Can you work these out from the drawing? Everything is in mm from the part's minimum corner. A direction names the side the tool comes from. Give positions to 0.01 mm unless a question says otherwise; leave off trailing zeros. Order: outer loops, then holes, each group sorted by start corner. A loop starts at its lowest first (then second) coordinate and runs counter-clockwise, first axis right, second up. Notation, with made-up numbers: M -33.5,74.5 L 7.5,74.5 A28 ccw 7.5,99.5 Z; hole C 47,67 d1. An arc over 180 degrees is marked long. Use a Markdown table: item, result. Add a question column.
Item 1: If I drill on L1, parallel to X at y = 1.55, z = 19.05; L2, parallel to Y at x = 24, z = 11.5; L3, parallel to Y at x = 5, z = 31.5, over which ranges is the centre line in solid material (lowest first)? Write a range as from..to.
Item 2: Suppose I cut it at D-D on x = 6.5. Write out the boundary of the cut face in (y, z).
Item 3: Suppose I cut it at B-B on y = 7.5. Write out the boundary of the cut face in (x, z).
Item 4: Suppose I cut it at C-C on z = 4. Write out the boundary of the cut face in (x, y).
Item 5: For the marked faces 4, 5 and 6, which set-ups out of +Z, -Z, +X, -X, +Y, -Y let a thin tool reach every point of the face, with its end or its side?
Item 6: I'm going to push flat-ended pins straight in: pin 1 Ø1 at (y, z) = (3, 4.5) entering from -X (1 decimal); pin 2 Ø1.5 at (x, z) = (6, 16) entering from -Y; pin 3 Ø3.5 at (x, y) = (20, 9.5) entering from +Z. Where does each tip first touch, or does it pass through?
Item 7: Suppose I cut it at A-A on x = 19.05. Write out the boundary of the cut face in (y, z).
Item 8: If we mould it in two halves opening along X, with no side actions, what happens to the marked faces 1, 2 and 3? For each: released by +X, released by -X, zero draft, split by the parting line, or undercut.
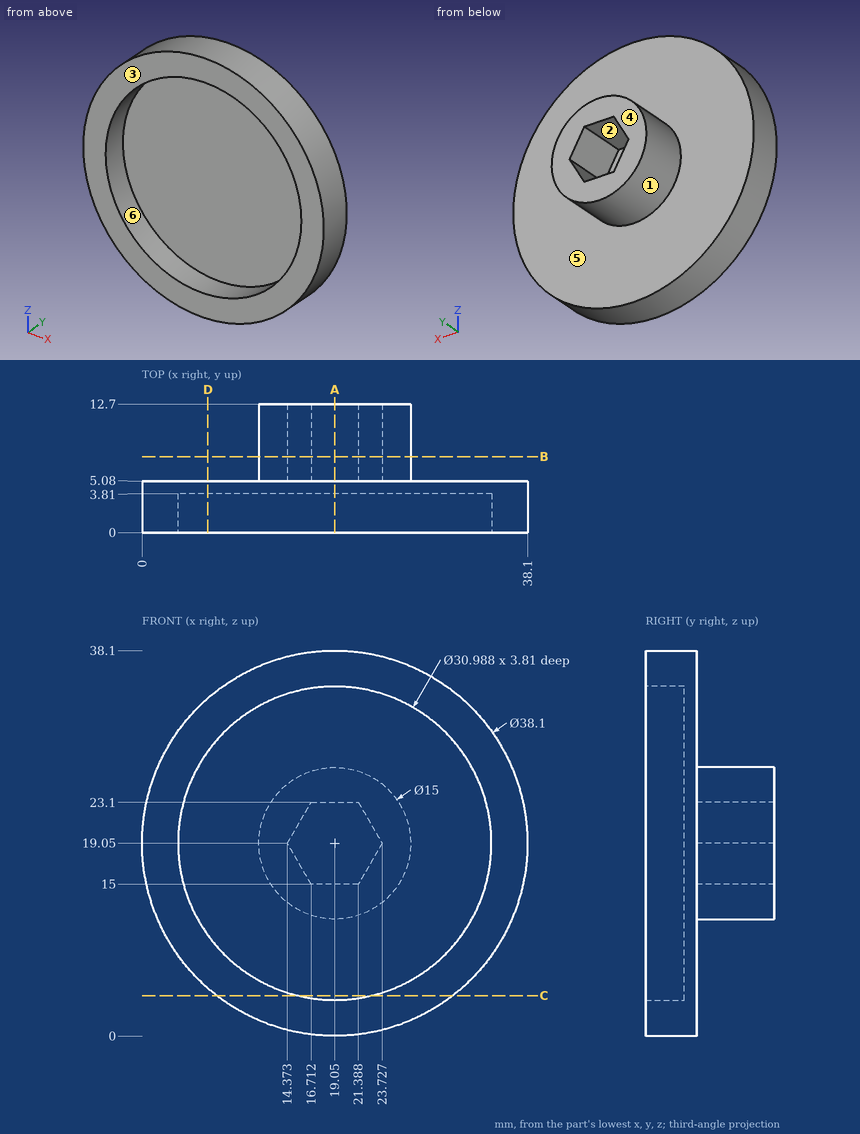
Findings below:
| question | item | result |
|---|---|---|
| 1 | L1 | x = 0..3.56, 34.54..38.1 |
| 1 | L2 | y = 3.81..5.08 |
| 1 | L3 | y = 0..5.08 |
| 2 | outline | M 0,4.72 L 5.08,4.72 L 5.08,33.38 L 0,33.38 L 0,28.14 L 3.81,28.14 L 3.81,9.96 L 0,9.96 Z |
| 3 | outline | C 19.05,19.05 d15; hole M 14.37,19.05 L 16.71,15 L 21.39,15 L 23.73,19.05 L 21.39,23.1 L 16.71,23.1 Z |
| 4 | outline | M 7.37,0 L 15.37,0 L 15.37,3.81 L 22.73,3.81 L 22.73,0 L 30.73,0 L 30.73,5.08 L 7.37,5.08 Z |
| 5 | face 4 | +Z, -Z, +X, -X, +Y |
| 5 | face 5 | +Y |
| 5 | face 6 | -Y |
| 6 | pin 1 | stops at x = 6.2 |
| 6 | pin 2 | stops at y = 3.81 |
| 6 | pin 3 | stops at z = 26.55 |
| 7 | outline | M 0,0 L 5.08,0 L 5.08,11.55 L 12.7,11.55 L 12.7,15 L 5.08,15 L 5.08,23.1 L 12.7,23.1 L 12.7,26.55 L 5.08,26.55 L 5.08,38.1 L 0,38.1 L 0,34.54 L 3.81,34.54 L 3.81,3.56 L 0,3.56 Z |
| 8 | face 1 | split by the parting line |
| 8 | face 2 | undercut |
| 8 | face 3 | zero draft |
